Verification items for the finished model (mm, model axes). Face numbers are marked on the shaded views. A direction names the side the tool comes from. Give positions to 0.01 mm unless a question says otherwise; leave off trailing zeros. Write each loop counter-clockwise with the first axis right and the second up, starting at its lowest first coordinate (ties: lowest second). Pieces come first, ordered by that corner, then holes. Notation, with made-up numbers: M 21,38.25 L 25,38.25 A35 ccw 25,76.25 Z; hole C 18.25,7 d10. An arc over 180 degrees is marked long. Answer as a JSON object with one key per item and string values.
Autodesk Inventor part; units mm, degrees
ref_plane "YZ Plane" through (0, 0, 0) normal (1, 0, 0) x (0, 1, 0)
ref_plane "XZ Plane" through (0, 0, 0) normal (0, 1, 0) x (-1, 0, 0)
ref_plane "XY Plane" through (0, 0, 0) normal (0, 0, 1) x (1, 0, 0)
sketch "Sketch1" plane through (0, 0, 0) normal (0, 0, 1) x (1, 0, 0)
  line L0 (-33.935, -38.575) -> (33.935, -38.575)
  line L1 (38.575, -33.935) -> (38.575, 33.935)
  line L2 (33.935, 38.575) -> (-33.935, 38.575)
  line L3 (-38.575, 33.935) -> (-38.575, -33.935)
  arc A0 (-33.935, 38.575) -> (-38.575, 33.935) centre (-33.935, 33.935) ccw
  arc A1 (38.575, 33.935) -> (33.935, 38.575) centre (33.935, 33.935) ccw
  arc A2 (-38.575, -33.935) -> (-33.935, -38.575) centre (-33.935, -33.935) ccw
  arc A3 (33.935, -38.575) -> (38.575, -33.935) centre (33.935, -33.935) ccw
  circle A4 centre (-30, 30) radius 2.55
  circle A5 centre (-10, 30) radius 2.1
  circle A6 centre (9.97, 30) radius 2.1
  circle A7 centre (30, 30) radius 2.55
  circle A8 centre (-30, 14.25) radius 3.6
  circle A9 centre (-20, 20) radius 2.1
  circle A10 centre (20, 20) radius 2.1
  circle A11 centre (0, 20) radius 2.55
  circle A12 centre (20, 10) radius 2.55
  circle A13 centre (-20, 10) radius 2.55
  circle A14 centre (-10, 10) radius 2.55
  circle A15 centre (0, 10) radius 2.55
  circle A16 centre (30, 14.25) radius 3.6
  circle A17 centre (-30, 0) radius 2.55
  circle A18 centre (-30, -14.25) radius 2.55
  circle A19 centre (-30, -30) radius 2.55
  circle A20 centre (9.97, 0) radius 2.55
  circle A21 centre (30, 0) radius 2.55
  line L4 (0, 0) -> (-10, 0) construction
  line L5 (0, 2.55) -> (-10, 2.55)
  line L6 (-10, -2.55) -> (0, -2.55)
  arc A22 (0, -2.55) -> (0, 2.55) centre (0, 0) ccw
  arc A23 (-10, 2.55) -> (-10, -2.55) centre (-10, 0) ccw
  circle A24 centre (-10, -30) radius 2.1
  circle A25 centre (9.97, -30) radius 2.1
  circle A26 centre (30, -30) radius 2.55
  circle A27 centre (-20, -20) radius 2.1
  circle A28 centre (20, -20) radius 2.1
  circle A29 centre (0, -20) radius 2.55
  circle A30 centre (20, -10) radius 2.55
  circle A31 centre (-20, -10) radius 2.55
  circle A32 centre (-10, -10) radius 2.55
  circle A33 centre (0, -10) radius 2.55
  circle A34 centre (30, -14.25) radius 2.55
  point P0 (0, 0)
  point P1 (38.575, 38.575)
  point P2 (38.575, -38.575)
  point P3 (-38.575, 38.575)
  point P4 (38.575, 0)
  point P5 (0, 38.575)
  point P6 (-5, 0)
  dimension "d0" = 77.15
  dimension "d1" = 77.15
  dimension "d2" = 4.64
  dimension "d3" = 5.1
  dimension "d4" = 4.2
  dimension "d5" = 8.575
  dimension "d6" = 18.575
  dimension "d7" = 8.575
  dimension "d8" = 7.2
  dimension "d9" = 24.325
  dimension "d10" = 38.575
  dimension "d11" = 52.825
  dimension "d12" = 68.575
  dimension "d13" = 28.575
  dimension "d14" = 18.575
  dimension "d15" = 38.575
  dimension "d16" = 48.545
  dimension "d17" = 58.575
  dimension "d18" = 68.575
  dimension "d19" = 28.575
  dimension "d20" = 10
  dimension "d21" = 5.1
  dimension "d22" = 5.1
extrude "Extrusion1" add sketch "Sketch1" along normal blind 6
sketch "Sketch2" plane through (0, 0, 6) normal (0, 0, 1) x (1, 0, 0)
  circle A0 centre (-30, 14.25) radius 3.6
  circle A1 centre (30, 14.25) radius 3.6
  circle A2 centre (-30, -14.25) radius 2.55
  circle A3 centre (30, -14.25) radius 2.55
  circle A4 centre (-30, 14.25) radius 6
  circle A5 centre (-30, -14.25) radius 4.5
  circle A6 centre (30, -14.25) radius 4.5
  circle A7 centre (30, 14.25) radius 6
  line L0 (-10.025, 14.945) -> (10.035, 14.945)
  line L1 (14.955, 10.025) -> (14.955, -10.035)
  line L2 (10.035, -14.955) -> (-10.025, -14.955)
  line L3 (-14.945, -10.035) -> (-14.945, 10.025)
  line L4 (-38.575, 33.935) -> (-38.575, -33.935)
  line L5 (33.935, 38.575) -> (-33.935, 38.575)
  arc A8 (-14.945, -10.035) -> (-10.025, -14.955) centre (-10.025, -10.035) ccw
  arc A9 (10.035, -14.955) -> (14.955, -10.035) centre (10.035, -10.035) ccw
  arc A10 (14.955, 10.025) -> (10.035, 14.945) centre (10.035, 10.025) ccw
  arc A11 (-10.025, 14.945) -> (-14.945, 10.025) centre (-10.025, 10.025) ccw
  point P0 (0, 0)
  dimension "d25" = 12
  dimension "d26" = 9
  dimension "d27" = 23.63
  dimension "d28" = 53.53
  dimension "d29" = 23.63
  dimension "d30" = 53.53
  dimension "d31" = 4.92
extrude "Extrusion2" cut sketch "Sketch2" against normal blind 1.5
thread "Thread1"
thread "Thread2"
thread "Thread3"
thread "Thread4"
thread "Thread5"
thread "Thread6"
thread "Thread7"
thread "Thread8"
properties part number "C-Beam Gantry Plate" material "Aluminum 6061"
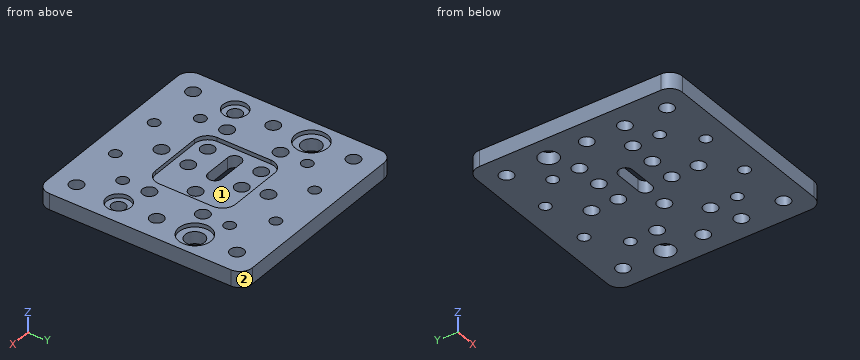
1) Section check C-C on y = -20. Record the boundary of the cut face in (x, z) (3 decimals).
Completed:
{"outline": "M -38.575,0 L -22.1,0 L -22.1,6 L -38.575,6 Z; M -17.9,0 L -2.55,0 L -2.55,6 L -17.9,6 Z; M 2.55,0 L 17.9,0 L 17.9,6 L 2.55,6 Z; M 22.1,0 L 38.575,0 L 38.575,6 L 22.1,6 Z"}
2) Thickness scan on L1, parallel to Y at x = -30, z = 0.9 (3 decimals); L2, parallel to Y at x = 9.97, z = 4.4 (3 decimals); L3, parallel to Y at x = 30, z = 5.6 (3 decimals). Record the ranges inside material, lowest first.
Completed:
{"L1": "y = -38.575 to -32.55, -27.45 to -16.8, -11.7 to -2.55, 2.55 to 10.65, 17.85 to 27.45, 32.55 to 38.575", "L2": "y = -38.575 to -32.1, -27.9 to -2.55, 2.55 to 27.9, 32.1 to 38.575", "L3": "y = -38.575 to -32.55, -27.45 to -18.75, -9.75 to -2.55, 2.55 to 8.25, 20.25 to 27.45, 32.55 to 38.575"}
3) Access from +Z, -Z, +X, -X, +Y, -Y to the whole of each face (thin tool, end or side, straight path). Record for the marked faces 1 and 2.
Completed:
{"face 1": "+Z", "face 2": "+Z, -Z, +X, +Y"}
4) Section check D-D on z = 1.9. Count the separate pieces of the cut face and the enclosed holes in it, and give its area (3 significant figures).
Completed:
{"separate pieces": "1", "enclosed holes": "30", "area": "5,280 mm2"}
5) Section check A-A on y = -30. Record the boundary of the cut face in (x, z) (3 decimals).
Completed:
{"outline": "M -38.575,0 L -32.55,0 L -32.55,6 L -38.575,6 Z; M -27.45,0 L -12.1,0 L -12.1,6 L -27.45,6 Z; M -7.9,0 L 7.87,0 L 7.87,6 L -7.9,6 Z; M 12.07,0 L 27.45,0 L 27.45,6 L 12.07,6 Z; M 32.55,0 L 38.575,0 L 38.575,6 L 32.55,6 Z"}
6) Go/stop test with flat-tipped pins: pin 1 (15 mm diameter, centred on x = 1.5, y = -1, fed in from +Z); pin 2 (4 mm diameter, centred on x = 30, y = -14.25, fed in from +Z). Record where each tip stops, or that it passes through.
Completed:
{"pin 1": "stops at z = 4.5", "pin 2": "passes through"}
7) Section check B-B on x = -20. Record the boundary of the cut face in (y, z) (3 decimals), and give its area (3 significant figures).
Completed:
{"outline": "M -38.575,0 L -22.1,0 L -22.1,6 L -38.575,6 Z; M -17.9,0 L -12.55,0 L -12.55,6 L -17.9,6 Z; M -7.45,0 L 7.45,0 L 7.45,6 L -7.45,6 Z; M 12.55,0 L 17.9,0 L 17.9,6 L 12.55,6 Z; M 22.1,0 L 38.575,0 L 38.575,6 L 22.1,6 Z", "area": "351 mm2"}
